from build123d import *

# Parameters (mm, degrees)
SKETCH1_W           = 50
SKETCH1_H           = 80
BOSS_EXTRUDE1_DEPTH = 42
SKETCH2_W           = 35
SKETCH2_H           = 45
BOSS_EXTRUDE2_DEPTH = 5
SKETCH3_R           = 4
CUT_EXTRUDE1_DEPTH  = 77.576758876


with BuildPart() as part:
    # Sketch1 → Boss-Extrude1 (new body)
    with BuildSketch(Plane(origin=(0, 0, 0), x_dir=(1, 0, 0), z_dir=(0, 1, 0))):
        Rectangle(SKETCH1_W, SKETCH1_H)
    extrude(amount=BOSS_EXTRUDE1_DEPTH)

    # Sketch2 → Boss-Extrude2 (add)
    with BuildSketch(Plane.XZ):
        Rectangle(SKETCH2_W, SKETCH2_H)
    extrude(amount=BOSS_EXTRUDE2_DEPTH)

    # Sketch3 → Cut-Extrude1 (cut, through all)
    with BuildSketch(Plane.ZY.offset(25)):
        with Locations((-30, 32)):
            Circle(SKETCH3_R)
        with Locations((30, 32)):
            Circle(SKETCH3_R)
    extrude(amount=-CUT_EXTRUDE1_DEPTH, mode=Mode.SUBTRACT)


solid = part.part
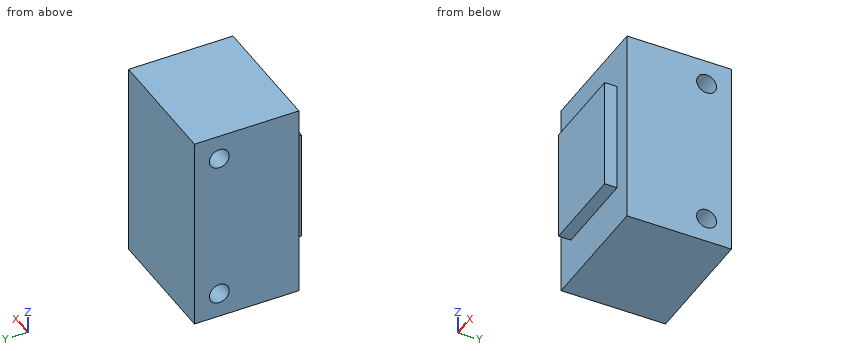
Design review of the part built by this model. Coordinates are the model's own, in mm. Round coordinates to 2 decimals unless told otherwise and drop trailing zeros. Loops run counter-clockwise (first coordinate to the right, second up) from the corner with the lowest first, then second, coordinate; pieces in that order, holes last. Notation, with made-up numbers: M 29.25,36.25 L 61.25,36.25 A7 ccw 61.25,49.25 Z; hole C 29.5,-22.75 d6. An arc over 180 degrees is marked long. Answer as a JSON object with one key per item and string values.
Item 1: We need section D-D on z = -10. Give the boundary of the cut face in (x, y), and give its area (4 significant figures).
Answer sheet:
{"outline": "M -25,0 L -17.5,0 L -17.5,-5 L 17.5,-5 L 17.5,0 L 25,0 L 25,42 L -25,42 Z", "area": "2,275 mm^2"}
Item 2: We need section B-B on y = 32. Give the boundary of the cut face in (x, z), and give its area (3 significant figures).
Answer sheet:
{"outline": "M -25,-40 L 25,-40 L 25,-34 L -25,-34 Z; M -25,-26 L 25,-26 L 25,26 L -25,26 Z; M -25,34 L 25,34 L 25,40 L -25,40 Z", "area": "3,200 mm^2"}
Item 3: Clearance check with flat-ended pins moving along their axes: P1, Ø1.5, axis at x = 6, y = -3, coming from the +Z side; P2, Ø1.5, axis at y = -3, z = -7, coming from the +X side. State where each tip first meets the part, or that it passes through.
Answer sheet:
{"P1": "stops at z = 22.5", "P2": "stops at x = 17.5"}
Item 4: We need section C-C on x = 9. Give the boundary of the cut face in (y, z), and give its area (3 significant figures).
Answer sheet:
{"outline": "M -5,-22.5 L 0,-22.5 L 0,-40 L 42,-40 L 42,40 L 0,40 L 0,22.5 L -5,22.5 Z; hole C 32,-30 d8; hole C 32,30 d8", "area": "3,480 mm^2"}
Item 5: Wall thickness on L1, parallel to Y at x = -13, z = -30; L2, parallel to Y at x = 2, z = 25; L3, parallel to Z at x = -3.5, y = 29.5: over which ranges is each line inside the solid? List them lowest first. Write a range as from..to.
Answer sheet:
{"L1": "y = 0..28, 36..42", "L2": "y = 0..42", "L3": "z = -40..-33.12, -26.88..26.88, 33.12..40"}
Item 6: We need section A-A on z = 30. Give the boundary of the cut face in (x, y).
Answer sheet:
{"outline": "M -25,0 L 25,0 L 25,28 L -25,28 Z; M -25,36 L 25,36 L 25,42 L -25,42 Z"}
